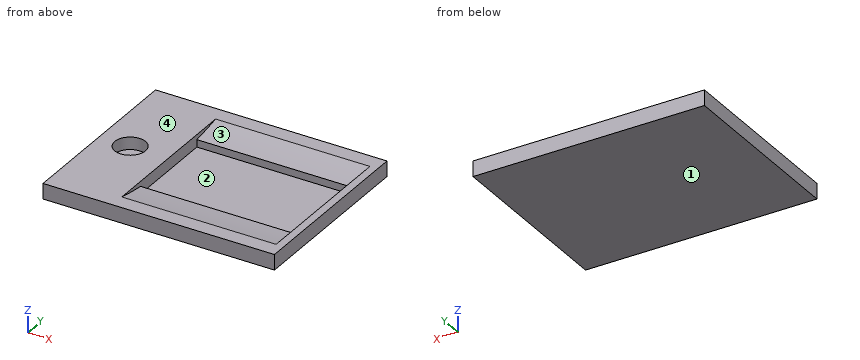
from build123d import *

# Parameters (mm, degrees)
SKETCH1_W           = 47.625
SKETCH1_H           = 38.1
BOSS_EXTRUDE1_DEPTH = 1.5875
SKETCH2_W           = 31.75
SKETCH2_H           = 19.05
SKETCH2_R           = 3.175
CUT_EXTRUDE1_DEPTH  = 2.54
CUT_EXTRUDE2_START  = -1.5875
CUT_EXTRUDE2_DEPTH  = 31.75


with BuildPart() as part:
    # Sketch1 → Boss-Extrude1 (new body, symmetric)
    with BuildSketch(Plane.XY):
        Rectangle(SKETCH1_W, SKETCH1_H)
    extrude(amount=BOSS_EXTRUDE1_DEPTH, both=True)

    # Sketch2 → Cut-Extrude1 (cut)
    with BuildSketch(Plane.XY.offset(1.5875)):
        with Locations((6.35, 0)):
            Rectangle(SKETCH2_W, SKETCH2_H)
        with Locations((-17.4625, 0)):
            Circle(SKETCH2_R)
    extrude(amount=-CUT_EXTRUDE1_DEPTH, mode=Mode.SUBTRACT)

    # Sketch4 → Cut-Extrude2 (cut)
    with BuildSketch(Plane(origin=(23.8125, 0, 0), x_dir=(0, 0, -1), z_dir=(1, 0, 0)).offset(CUT_EXTRUDE2_START)):
        with BuildLine():
            ThreePointArc((0, 0), (-0.397862257, 7.977088774), (-1.5875, 15.875))
            Line((-1.5875, 15.875), (-1.5875, -15.875))
            ThreePointArc((-1.5875, -15.875), (-0.397862257, -7.977088774), (0, 0))
        make_face()
    extrude(amount=-CUT_EXTRUDE2_DEPTH, mode=Mode.SUBTRACT)


solid = part.part
Check sheet for the modelled part. Datum: model origin and axes. Units: mm. Face numbers are marked on the shaded views. A direction names the side the tool comes from. Round coordinates to 2 decimals unless told otherwise and drop trailing zeros. Order: outer loops, then holes, each group sorted by start corner. A loop starts at its lowest first (then second) coordinate and runs counter-clockwise, first axis right, second up.
(1) Draft check along X on the marked faces 1 and 2. Enter one of: pulls with the +X half, pulls with the -X half, needs draft (parallel to the pull), parting line crosses it, or undercut.
(2) Cross-section at C-C, the plane y = 0. Enter the section's corners in (x, z) (1 decimal), and give its area (3 significant figures).
(3) Go/stop test with a flat-tipped pin: P1, Ø8, axis at x = 11.5, y = -0.5, coming from the +Z side. Record where the tip stops, or that it passes through.
(4) Cross-section at D-D, the plane x = -18. Enter the section's corners in (y, z), and give its area (3 significant figures).
(5) Scan lines: probe 1 along X at (y, z) = (7, 0.3) (1 decimal); probe 2 along X at (y, z) = (-1, 0.6) (1 decimal); probe 3 along Y at (x, z) = (-3, -0.3) (3 decimals). Record each from-to range of solid material in increasing order.
(6) Cross-section at A-A, the plane z = -0.2. State how many separate pieces and enclosed holes the cut face has, and give its area (3 significant figures).
(7) Access from +Z, -Z, +X, -X, +Y, -Y to the whole of each face (thin tool, end or side, straight path). Record for the marked faces 3 and 4.
Check sheet entries:
1. face 1: needs draft
1. face 2: undercut
2. outline: (-23.8, -1.6) - (23.8, -1.6) - (23.8, 1.6) - (22.2, 1.6) - (22.2, -1) - (-9.5, -1) - (-9.5, 1.6) - (-14.3, 1.6) - (-14.3, -1) - (-20.6, -1) - (-20.6, 1.6) - (-23.8, 1.6) - close
2. area: 54.4 mm2
3. P1: stops at z = -0.95
4. outline: (-19.05, -1.59) - (19.05, -1.59) - (19.05, 1.59) - (3.13, 1.59) - (3.13, -0.95) - (-3.13, -0.95) - (-3.13, 1.59) - (-19.05, 1.59) - close
4. area: 105 mm2
5. probe 1: x = -23.8 to -9.5, 22.2 to 23.8
5. probe 2: x = -23.8 to -20.5, -14.4 to -9.5, 22.2 to 23.8
5. probe 3: y = -19.05 to -9.525, 9.525 to 19.05
6. separate pieces: 1
6. enclosed holes: 2
6. area: 1,180 mm2
7. face 3: +Z
7. face 4: +Z, +X, -X, +Y, -Y
